Source: CAD feature listing. Evaluate the final solid. Frame: model axes, mm. Round coordinates to 2 decimals unless told otherwise and drop trailing zeros. Write each loop counter-clockwise with the first axis right and the second up, starting at its lowest first coordinate (ties: lowest second). Pieces come first, ordered by that corner, then holes. Notation, with made-up numbers: M 25,-36.5 L 42,-36.5 A29 cw 42,-3.5 Z; hole C 72,60.25 d4. An arc over 180 degrees is marked long. Answer in a Markdown table with one row per item.
from build123d import *

# Parameters (mm, degrees)
BOSS_EXTRUDE1_DEPTH = 40.64
SKETCH6_R           = 1.1303
CUT_EXTRUDE1_DEPTH  = 158.779215984
SKETCH7_W           = 73.663303239
SKETCH7_H           = 73.66330324
CUT_EXTRUDE2_DEPTH  = 158.779215984
SKETCH8_R           = 1.1303
CUT_EXTRUDE3_DEPTH  = 145.040213208


with BuildPart() as part:
    # Sweep3: sweep along a path in Sketch2
    with BuildLine(Plane.XY) as sweep3_path:
        Line((-111.378641457, -46.568583299), (-11.322173751, -64.21123815))
        ThreePointArc((-11.322173751, -64.21123815), (49.947476571, -41.910909169), (61.269650322, 22.300328981))
        Line((61.269650322, 22.300328981), (48.238682861, 58.102617833))
    # 3DSketch1 → Sweep3 (sweep)
    with BuildSketch(Plane(origin=(-117.024291009, -78.586652965, -20.32), x_dir=(0.051794909001673446, 0.2937435257699459, 0.9544799780350292), z_dir=(0.984807753012208, -0.17364817766693055, 0))):
        Polygon((0, 0), (3.788092413, -12.121895721), (42.57815872, 0), (38.790066307, 12.121895721), align=None)
    sweep(path=sweep3_path.line)

    # Sketch5 → Boss-Extrude1 (add)
    with BuildSketch(Plane.XY.offset(20.32)):
        with BuildLine():
            Line((-16.967823303, -96.229307816), (-117.024291009, -78.586652965))
            Line((-117.024291009, -78.586652965), (-117.024291009, -97.7138))
            Line((-117.024291009, -97.7138), (-2e-08, -97.7138))
            ThreePointArc((-2e-08, -97.7138), (-8.516318826, -97.34196949), (-16.967823303, -96.229307816))
        make_face()
        with BuildLine():
            ThreePointArc((97.7138, 6e-08), (69.09409061, -69.094090581), (-2e-08, -97.7138))
            Line((-2e-08, -97.7138), (97.7138, -97.7138))
            Line((97.7138, -97.7138), (97.7138, 6e-08))
        make_face()
        with BuildLine():
            ThreePointArc((91.820936809, 33.420087881), (96.229307811, 16.967823332), (97.7138, 6e-08))
            Line((97.7138, 6e-08), (97.7138, 69.222376733))
            Line((97.7138, 69.222376733), (78.789969348, 69.222376733))
            Line((78.789969348, 69.222376733), (91.820936809, 33.420087881))
        make_face()
    extrude(amount=-BOSS_EXTRUDE1_DEPTH)

    # Sketch6 → Cut-Extrude1 (cut, through all)
    with BuildSketch(Plane.XY.offset(20.32)):
        with Locations((91.3638, -91.3638)):
            Circle(SKETCH6_R)
        with Locations((-41.9735, -91.3638)):
            Circle(SKETCH6_R)
    extrude(amount=-CUT_EXTRUDE1_DEPTH, mode=Mode.SUBTRACT)

    # Sketch7 → Cut-Extrude2 (cut, through all)
    with BuildSketch(Plane.XY.offset(20.32)):
        with Locations((-90.355942629, -60.88214838)):
            Rectangle(SKETCH7_W, SKETCH7_H)
    extrude(amount=-CUT_EXTRUDE2_DEPTH, mode=Mode.SUBTRACT)

    # Sketch8 → Cut-Extrude3 (cut, through all)
    with BuildSketch(Plane.XY.offset(20.32)):
        with Locations((-47.174291009, -91.3638)):
            Circle(SKETCH8_R)
    extrude(amount=-CUT_EXTRUDE3_DEPTH, mode=Mode.SUBTRACT)


solid = part.part
Q1. Material intervals for probe 1 along X at (y, z) = (-1.5, 6); probe 2 along X at (y, z) = (16.5, 8); probe 3 along Y at (x, z) = (12, -18), sorted ascending.
Solutions:
| item | result |
|---|---|
| probe 1 | x = 85 to 97.71 |
| probe 2 | x = 83.4 to 97.71 |
| probe 3 | y = -97.71 to -84.16 |
Q2. Section D-D (x = -21). Return loops of the section in (y, z), and give its area (3 significant figures).
Solutions:
| item | result |
|---|---|
| outline | M -97.71,-20.32 L -82.62,-20.32 L -82.62,20.32 L -97.71,20.32 Z |
| area | 613 mm2 |
Q3. Section B-B (x = 75). Return loops of the section in (y, z), and give its area (3 significant figures).
Solutions:
| item | result |
|---|---|
| outline | M -97.71,-20.32 L -40.03,-20.32 L -40.03,20.32 L -97.71,20.32 Z; M 42.5,-20.32 L 67.84,-20.32 L 67.84,20.32 L 42.5,20.32 Z |
| area | 3,370 mm2 |
Q4. Section C-C (z = -6). Return loops of the section in (x, y).
Solutions:
| item | result |
|---|---|
| outline | M -53.52,-97.71 L 97.71,-97.71 L 97.71,69.22 L 78.79,69.22 L 66.86,64.88 L 79.89,29.08 A85.01 cw -14.76,-83.72 L -53.52,-76.89 Z; hole C -47.17,-91.36 d2.26; hole C -41.97,-91.36 d2.26; hole C 91.36,-91.36 d2.26 |
Q5. Section A-A (y = -81.5). Return loops of the section in (x, z), and give its area (3 significant figures).
Solutions:
| item | result |
|---|---|
| outline | M -53.52,-20.32 L -27.37,-20.32 L -27.37,20.32 L -53.52,20.32 Z; M 24.19,-20.32 L 97.71,-20.32 L 97.71,20.32 L 24.19,20.32 Z |
| area | 4,050 mm2 |
Q6. Contact query for flat-ended pins moving along their axis: pin 1 Ø1.4 at (x, y) = (-47.17, -91.36) entering from +Z; pin 2 Ø1.5 at (y, z) = (-29, 9.5) entering from -X. Output: stop coordinate, or through.
Solutions:
| item | result |
|---|---|
| pin 1 | passes through |
| pin 2 | stops at x = 79.64 |
Q7. Pull-direction query (X, two-part tool) for faces 1 (the flat face through (-33.872, -80.353, -0.284)), 2 (the flat face through (73.28, 47.23, -0.28)), 3 (the flat face through (21, -97.714, 0)); classes: pulls with the +X half, pulls with the -X half, needs draft (parallel to the pull), parting line crosses it, or undercut.
Solutions:
| item | result |
|---|---|
| face 1 | undercut |
| face 2 | pulls with the -X half |
| face 3 | needs draft |
